Job drawing, mm, ordinate dimensions from the low corner. One solid piece. A direction names the side the tool comes from. Give positions to 0.01 mm unless a question says otherwise; leave off trailing zeros. Order: outer loops, then holes, each group sorted by start corner. A loop starts at its lowest first (then second) coordinate and runs counter-clockwise, first axis right, second up. Notation, with made-up numbers: M -39,-19.5 L -10,-19.5 A32 cw -10,8.5 Z; hole C -19,58.5 d1. An arc over 180 degrees is marked long. Put each result on its own line as item: value. Start each with the question number.
1) Pin check, flat tips, straight feed: pin 1 (5 mm diameter, centred on x = 87.5, z = 30, fed in from -Y); pin 2 (9 mm diameter, centred on x = 100.8, y = 20, fed in from -Z); pin 3 (4.5 mm diameter, centred on x = 10, y = 20, fed in from +Z); pin 4 (5 mm diameter, centred on x = 42.5, y = 18.5, fed in from -Z). Stop position of each tip, or through.
2) Cut at B-B (x = 100.8). Write the cut outline in (y, z), and give its area (3 significant figures).
3) Cut at C-C (z = 26.5). Write the cut outline in (x, y).
4) Drill centre lines: line 1 (Y direction, x = 10, z = 31); line 2 (X direction, y = 23.5, z = 25.5); line 3 (X direction, y = 34.5, z = 33). Where is each one in solid material? Low to high. Write a range as [from, to].
5) Two-plate mould, pull along X, no slides. Class the marked faces 1, 2 and 3: released by +X, released by -X, zero draft, split by the parting line, or undercut.
6) Cut at D-D (z = 15.5). Write the cut outline in (x, y), and give its area (3 significant figures).
7) Tool access for the marked faces 4, 5 and 6: list every direction of +Z, -Z, +X, -X, +Y, -Y with a clear straight run to the whole face (end or side of a thin tool).
8) Cut at A-A (y = 20). Write the cut outline in (x, z).
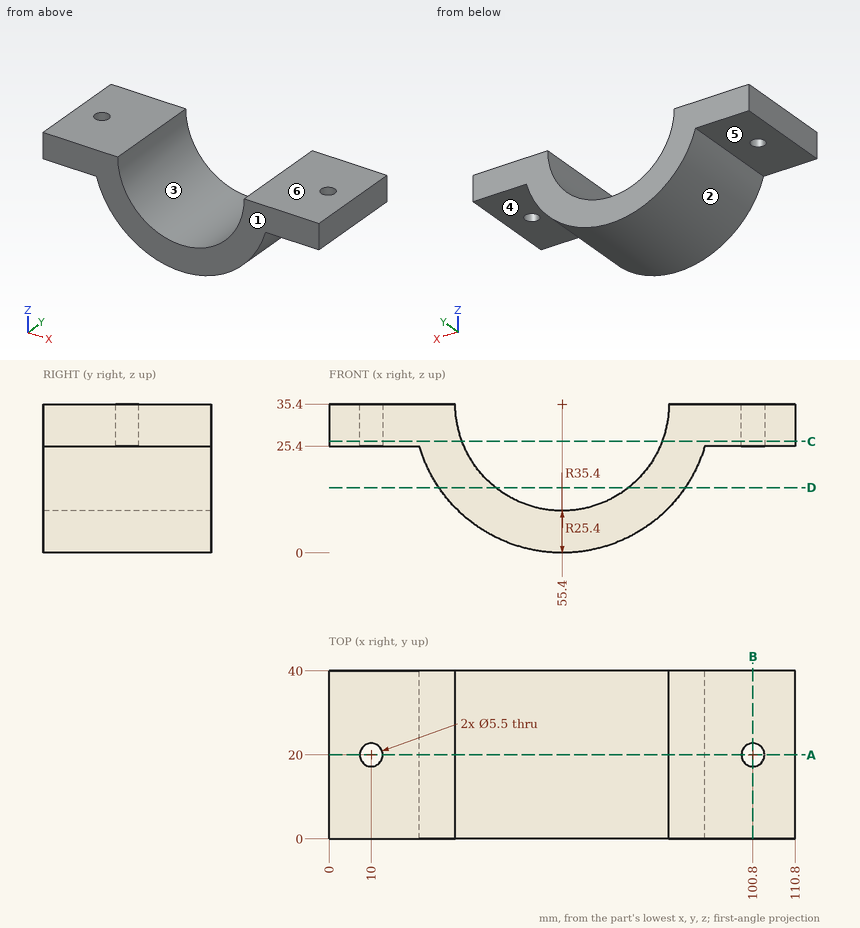
Solution:
1. pin 1: y = 0
1. pin 2: z = 25.4
1. pin 3: through
1. pin 4: z = 1.56
2. outline: M 0,25.4 L 17.25,25.4 L 17.25,35.4 L 0,35.4 Z; M 22.75,25.4 L 40,25.4 L 40,35.4 L 22.75,35.4 Z
2. area: 345 mm²
3. outline: M 0,0 L 31.61,0 L 31.61,40 L 0,40 Z; M 79.19,0 L 110.8,0 L 110.8,40 L 79.19,40 Z; hole C 10,20 d5.5; hole C 100.8,20 d5.5
4. line 1: [0, 17.25], [22.75, 40]
4. line 2: [0, 32.01], [78.79, 110.8]
4. line 3: [0, 30.11], [80.69, 110.8]
5. face 1: zero draft
5. face 2: split by the parting line
5. face 3: undercut
6. outline: M 26.12,0 L 39.62,0 L 39.62,40 L 26.12,40 Z; M 71.18,0 L 84.68,0 L 84.68,40 L 71.18,40 Z
6. area: 1,080 mm²
7. face 4: -Z, +X, +Y, -Y
7. face 5: -Z, -X, +Y, -Y
7. face 6: +Z, +X, -X, +Y, -Y
8. outline: M 0,25.4 L 7.25,25.4 L 7.25,35.4 L 0,35.4 Z; M 12.75,25.4 L 21.44,25.4 A35.4 ccw 89.36,25.4 L 98.05,25.4 L 98.05,35.4 L 80.8,35.4 A25.4 cw 30,35.4 L 12.75,35.4 Z; M 103.55,25.4 L 110.8,25.4 L 110.8,35.4 L 103.55,35.4 Z
